Geometry check sheet. Reference: the model listing, model coordinates, mm. A direction names the side the tool comes from. Coordinates: 2 decimals unless noted, no trailing zeros. Write each loop counter-clockwise with the first axis right and the second up, starting at its lowest first coordinate (ties: lowest second). Pieces come first, ordered by that corner, then holes. Notation, with made-up numbers: (20.5, 42.25) -> (62.5, 42.25) arc R25 cw to (62.5, 59.25) -> close; hole circle Ø10 at (47, -35). An arc over 180 degrees is marked (long way). Answer in a Markdown table with one row per item. Add a question column.
1. Cross-section at A-A on x = 0. Record the cut outline in (y, z), and give its area (3 significant figures).
2. Scan lines: L1, parallel to Z at x = 2.2, y = -0.35; L2, parallel to Y at x = 0, z = -1; L3, parallel to X at y = -0.55, z = -1.5. Record each from-to range of solid material in increasing order. Write a range as from..to.
3. Depth check by flat-ended pin: P1, Ø1, axis at y = 0, z = -1.5, coming from the +X side; P2, Ø3, axis at x = -1.5, z = -2.5, coming from the +Y side; P3, Ø2, axis at y = 1.5, z = -0.5, coming from the +X side. Enter the tip coordinate at first touch or a pass-through.
4. Set-up check for faces 1 (the flat face through (-1, -1, 0)), 2 (the flat face through (0, 0, 2)): record each of +Z, -Z, +X, -X, +Y, -Y from which the full face is reachable in a straight line by a thin tool's end or side.
5. Cross-section at D-D on x = 2. Record the cut outline in (y, z), and give its area (3 significant figures).
6. Cross-section at C-C on z = 1.5. Record the cut outline in (x, y), and give its area (3 significant figures).
```python
from build123d import *

# Parameters (mm, degrees)
CROQUIS1_R              = 2.5
SALIENTE_EXTRUIR1_DEPTH = 2
CROQUIS2_R              = 1.2
SALIENTE_EXTRUIR2_DEPTH = 6
CHAFL_N1_SIZE           = 0.5
CHAFL_N1_SIZE2          = 0.866025404


with BuildPart() as part:
    # Croquis1 → Saliente-Extruir1 (new body)
    with BuildSketch(Plane.XY):
        Circle(CROQUIS1_R)
    extrude(amount=SALIENTE_EXTRUIR1_DEPTH)

    # Croquis2 → Saliente-Extruir2 (add)
    with BuildSketch(Plane.XY):
        Circle(CROQUIS2_R)
    extrude(amount=-SALIENTE_EXTRUIR2_DEPTH)

    # Chaflán1
    chafl_n1_edges = [part.edges().sort_by_distance(p)[0] for p in [
        (-1.2, 0, -6),
    ]]
    chafl_n1_side = [part.faces().sort_by_distance(p)[0] for p in [
        (0, 0, -6),
    ]]
    chamfer(chafl_n1_edges, length=CHAFL_N1_SIZE, length2=CHAFL_N1_SIZE2, reference=chafl_n1_side[0])


solid = part.part
```
Results found:
| question | item | result |
|---|---|---|
| 1 | outline | (-2.5, 0) -> (-1.2, 0) -> (-1.2, -5.13) -> (-0.7, -6) -> (0.7, -6) -> (1.2, -5.13) -> (1.2, 0) -> (2.5, 0) -> (2.5, 2) -> (-2.5, 2) -> close |
| 1 | area | 24.0 mm^2 |
| 2 | L1 | z = 0..2 |
| 2 | L2 | y = -1.2..1.2 |
| 2 | L3 | x = -1.07..1.07 |
| 3 | P1 | stops at x = 1.2 |
| 3 | P2 | stops at y = 1.2 |
| 3 | P3 | stops at x = 2.42 |
| 4 | face 1 | -Z |
| 4 | face 2 | +Z, +X, -X, +Y, -Y |
| 5 | outline | (-1.5, 0) -> (1.5, 0) -> (1.5, 2) -> (-1.5, 2) -> close |
| 5 | area | 6.00 mm^2 |
| 6 | outline | circle Ø5 at (0, 0) |
| 6 | area | 19.6 mm^2 |
